Here's how the part is built. I have some questions about the finished solid (model axes, mm). A direction names the side the tool comes from. Round coordinates to 2 decimals unless told otherwise and drop trailing zeros. Write each loop counter-clockwise with the first axis right and the second up, starting at its lowest first coordinate (ties: lowest second). Pieces come first, ordered by that corner, then holes. Notation, with made-up numbers: (-31.5, -35) -> (3.5, -35) arc R24 cw to (3.5, 0) -> close; hole circle Ø10 at (84, -34.75). An arc over 180 degrees is marked (long way). Answer in a Markdown table with one row per item.
from build123d import *

# Parameters (mm, degrees)
F0_W     = 7.5
F0_H     = 10.3
F1_DEPTH = 2.3
F2_W     = 1.4
F2_H     = 0.4
F3_DEPTH = 0.99318
F5_COUNT = 2
F5_ANGLE = 180


with BuildPart() as f1:
    # F0 (on Top) → F1 (new body)
    with BuildSketch(Plane.XY):
        Rectangle(F0_W, F0_H)
    extrude(amount=F1_DEPTH)

    # F2 (on Top) → F3 (join)
    with BuildSketch(Plane.XY):
        with Locations((-4.45, 4.445)):
            Rectangle(F2_W, F2_H)
        with Locations((-4.45, 3.175)):
            Rectangle(F2_W, F2_H)
        with Locations((-4.45, 1.905)):
            Rectangle(F2_W, F2_H)
        with Locations((-4.45, -1.905)):
            Rectangle(F2_W, F2_H)
        with Locations((-4.45, 0.635)):
            Rectangle(F2_W, F2_H)
        with Locations((-4.45, -0.635)):
            Rectangle(F2_W, F2_H)
        with Locations((-4.45, -3.175)):
            Rectangle(F2_W, F2_H)
        with Locations((-4.45, -4.445)):
            Rectangle(F2_W, F2_H)
    extrude(amount=F3_DEPTH)

    # F5: F1 ×2 about axis
    f5_axis = Axis((0, 0, 4.798143), (0, 0, 1))


with BuildPart() as f1_1:
    add(f1.part)
    for i in range(1, F5_COUNT):
        add(f1.part.rotate(f5_axis, i * F5_ANGLE / (F5_COUNT - 1)))


solid = f1_1.part
1) I need wall thicknesses on line 1 (X direction, y = 0, z = 0.5); line 2 (Z direction, x = -4, y = 1.75). Which ranges of each line are inside material? Lowest first, please. Write a range as [from, to].
Response:
| item | result |
|---|---|
| line 1 | x = [-3.75, 3.75] |
| line 2 | z = [0, 0.99] |
2) We'd pull the mould along Y, two halves only. Please class faces 1 (the face through (-4.5, -2.975, 0.5)), 2 (the face through (0, 5.15, 1)), 3 (the face through (-4.5, -4.645, 0.5)), 4 (the face through (-4.5, 2.975, 0.5)): +Y half, -Y half, draft (parallel to the pull), parting line (faces both ways), or undercut.
Response:
| item | result |
|---|---|
| face 1 | undercut |
| face 2 | +Y half |
| face 3 | -Y half |
| face 4 | undercut |
3) I want a section at A-A, the plane z = 1.6. List the corners of the cut face in (x, y) for me, and give its area (4 significant figures).
Response:
| item | result |
|---|---|
| outline | (-3.75, -5.15) -> (3.75, -5.15) -> (3.75, 5.15) -> (-3.75, 5.15) -> close |
| area | 77.25 mm^2 |
4) I want a section at B-B, the plane y = 0. List the corners of the cut face in (x, z) for me, and give its area (4 significant figures).
Response:
| item | result |
|---|---|
| outline | (-3.75, 0) -> (3.75, 0) -> (3.75, 2.3) -> (-3.75, 2.3) -> close |
| area | 17.25 mm^2 |
5) For pin 1 (0.8 mm diameter, centred on x = -4.5, z = 0.5, fed in from -Y) (3 decimals); pin 2 (1.1 mm diameter, centred on x = -4.5, z = 0.5, fed in from +Y) (3 decimals), each with a flat end and sliding along its axis, tell me the tip position at first contact or that it passes through.
Response:
| item | result |
|---|---|
| pin 1 | stops at y = -4.645 |
| pin 2 | stops at y = 4.645 |
6) Which directions (+Z, -Z, +X, -X, +Y, -Y) give clear straight access to the entire face, cutting with the end or side of a thin tool? Please do faces 5 (the face through (4.5, 0.835, 0.5)), 6 (the face through (0, -5.15, 1)), 7 (the face through (-4.5, -1.705, 0.5)), 8 (the face through (4.5, -4.645, 0.5)).
Response:
| item | result |
|---|---|
| face 5 | +Z, -Z, +X |
| face 6 | +Z, -Z, +X, -X, -Y |
| face 7 | +Z, -Z, -X |
| face 8 | +Z, -Z, +X, -Y |
